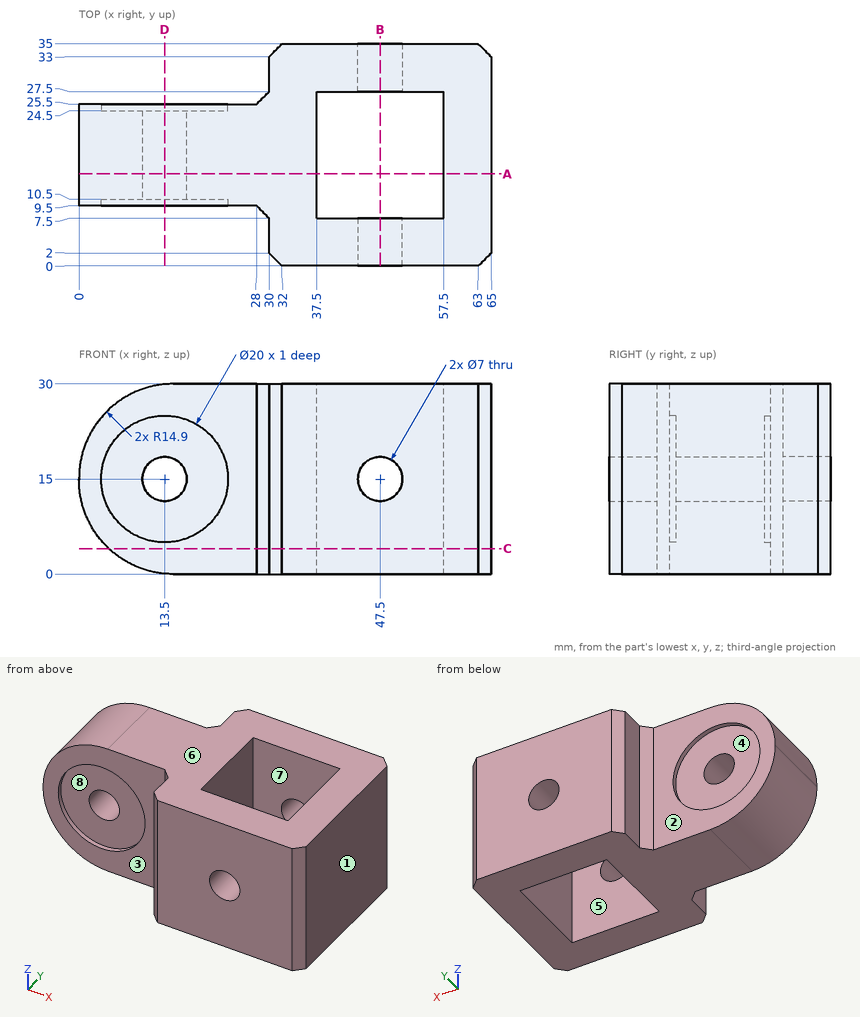
Can you work these out from the drawing? Everything is in mm from the part's minimum corner. A direction names the side the tool comes from. Coordinates: 2 decimals unless noted, no trailing zeros. Order: outer loops, then holes, each group sorted by start corner. A loop starts at its lowest first (then second) coordinate and runs counter-clockwise, first axis right, second up. Notation, with made-up numbers: (10.25, -6) -> (64.25, -6) arc R20 cw to (64.25, 3) -> close; hole circle Ø1 at (-2, 4.5). An arc over 180 degrees is marked (long way). Return JSON: item names as keys, results as strings.
1) Thinking about a two-plate mould opening in Y: for the marked faces 6, 7 and 8, which applies, +Y half, -Y half, draft (parallel to the pull), parting line (faces both ways), or undercut?
Conclusion:
{"face 6": "draft", "face 7": "undercut", "face 8": "-Y half"}
2) If we section it at A-A on y = 14.5: List the corners of the cut face in (x, z) for me, plus the area to 3 significant figures.
Conclusion:
{"outline": "(0, 14.9) arc R14.9 ccw to (14.9, 0) -> (37.5, 0) -> (37.5, 30) -> (14.9, 30) arc R14.9 ccw to (0, 15.1) -> close; (57.5, 0) -> (65, 0) -> (65, 30) -> (57.5, 30) -> close; hole circle Ø7 at (13.5, 15)", "area": "1,220 mm²"}
3) If we section it at D-D on x = 13.5: List the corners of the cut face in (y, z) for me, plus the area to 3 significant figures.
Conclusion:
{"outline": "(9.5, 0.07) -> (25.5, 0.07) -> (25.5, 5) -> (24.5, 5) -> (24.5, 11.5) -> (10.5, 11.5) -> (10.5, 5) -> (9.5, 5) -> close; (9.5, 25) -> (10.5, 25) -> (10.5, 18.5) -> (24.5, 18.5) -> (24.5, 25) -> (25.5, 25) -> (25.5, 29.93) -> (9.5, 29.93) -> close", "area": "340 mm²"}
4) If I drill on probe 1 along Y at (x, z) = (47.5, 4.5); probe 2 along Z at (x, y) = (47.5, 30); probe 3 along X at (y, z) = (13.5, 17.5), over which ranges is the centre line in solid material (lowest first)?
Conclusion:
{"probe 1": "y = 0 to 7.5, 27.5 to 35", "probe 2": "z = 0 to 11.5, 18.5 to 30", "probe 3": "x = 0.19 to 11.05, 15.95 to 37.5, 57.5 to 65"}
5) If we section it at B-B on x = 47.5: List the corners of the cut face in (y, z) for me, plus the area to 3 significant figures.
Conclusion:
{"outline": "(0, 0) -> (7.5, 0) -> (7.5, 11.5) -> (0, 11.5) -> close; (0, 18.5) -> (7.5, 18.5) -> (7.5, 30) -> (0, 30) -> close; (27.5, 0) -> (35, 0) -> (35, 11.5) -> (27.5, 11.5) -> close; (27.5, 18.5) -> (35, 18.5) -> (35, 30) -> (27.5, 30) -> close", "area": "345 mm²"}
6) On a 3-axis mill with a long thin cutter (end or side, diameter ignored), from which of +Z, -Z, +X, -X, +Y, -Y can I reach the whole of each face in a straight line? I mean the marked faces 1, 2, 3, 4 and 5. Say none if no direction works.
Conclusion:
{"face 1": "+Z, -Z, +X, +Y, -Y", "face 2": "+Z, -Z, -X, +Y", "face 3": "+Z, -Z, -X, -Y", "face 4": "+Y", "face 5": "+Z, -Z"}
7) I'm going to push flat-ended pins straight in: P1, Ø5, axis at y = 20, z = 23.5, coming from the -X side; P2, Ø6, axis at y = 29.5, z = 15.5, coming from the -X side; P3, Ø9, axis at x = 13.5, z = 15, coming from the +Y side; P4, Ø4, axis at x = 47.5, z = 15, coming from the -Y side. Where does each tip first touch, or does it pass through?
Conclusion:
{"P1": "stops at x = 1.22", "P2": "stops at x = 29", "P3": "stops at y = 24.5", "P4": "passes through"}
8) If we section it at C-C on z = 4: List the corners of the cut face in (x, y) for me.
Conclusion:
{"outline": "(4.74, 9.5) -> (28, 9.5) -> (30, 7.5) -> (30, 2) -> (32, 0) -> (63, 0) -> (65, 2) -> (65, 33) -> (63, 35) -> (32, 35) -> (30, 33) -> (30, 27.5) -> (28, 25.5) -> (4.74, 25.5) -> close; hole (37.5, 7.5) -> (57.5, 7.5) -> (57.5, 27.5) -> (37.5, 27.5) -> close"}
